```python
from build123d import *

# Parameters (mm, degrees)
PAD_DEPTH       = 250
SKETCH001_R     = 1.5
POCKET_DEPTH    = 10
SKETCH002_R     = 1.5
POCKET001_DEPTH = 10


with BuildPart() as part:
    # Sketch → Pad (new body)
    with BuildSketch(Plane.YZ):
        with BuildLine():
            Line((0, 0), (14, 0))
            Line((14, 0), (14, 1.524))
            Line((14, 1.524), (15.121, 1.524))
            Line((15.121, 1.524), (15.121, 7.862))
            ThreePointArc((15.121, 7.862), (8.692711, 6.292749), (2.787425, 3.307276))
            Line((0.963795, 6), (2.787425, 3.307276))
            Line((0, 6), (0.963795, 6))
            Line((0, 0), (0, 6))
        make_face()
    extrude(amount=PAD_DEPTH)

    # Sketch001 (on Face10 of Pad) → Pocket (cut)
    with BuildSketch(Plane.YZ.offset(250)):
        with Locations((12, 4)):
            Circle(SKETCH001_R)
        with Locations((5, 2)):
            Circle(SKETCH001_R)
    extrude(amount=-POCKET_DEPTH, mode=Mode.SUBTRACT)

    # Sketch002 (on Face4 of Pocket) → Pocket001 (cut)
    with BuildSketch(Plane(origin=(0, 0, 0), x_dir=(0, 1, 0), z_dir=(-1, 0, 0))):
        with Locations((12, -4)):
            Circle(SKETCH002_R)
        with Locations((5, -2)):
            Circle(SKETCH002_R)
    extrude(amount=-POCKET001_DEPTH, mode=Mode.SUBTRACT)


solid = part.part
```
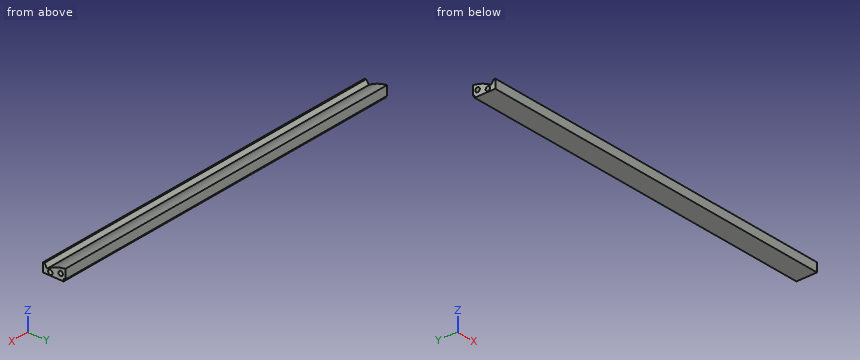
Work out the finished part from the listing and answer in its coordinate system (mm). Give positions to 0.01 mm unless a question says otherwise; leave off trailing zeros. Order: outer loops, then holes, each group sorted by start corner. A loop starts at its lowest first (then second) coordinate and runs counter-clockwise, first axis right, second up. Notation, with made-up numbers: M -3.75,25.5 L 3.25,25.5 A29 ccw 3.25,61.5 Z; hole C 18,-33 d4. An arc over 180 degrees is marked long. Return JSON: item names as keys, results as strings.
1) Straight lines are drawn through the part: line 1 along Y through (x, z) = (8.25, 2); line 2 along Y through (x, z) = (4.75, 4); line 3 along Z through (x, y) = (245.5, 5). For each, find the intervals that lie inside material, in ascending order. Write a range as [from, to].
Resolved:
{"line 1": "[0, 3.5], [6.5, 15.12]", "line 2": "[0, 2.32], [3.89, 10.5], [13.5, 15.12]", "line 3": "[0, 0.5], [3.5, 4.63]"}
2) Section A-A, the plane x = 148 is taken. Write down the section's boundary in (y, z), plus the area to 3 significant figures.
Resolved:
{"outline": "M 0,0 L 14,0 L 14,1.52 L 15.12,1.52 L 15.12,7.86 A29 ccw 2.79,3.31 L 0.96,6 L 0,6 Z", "area": "88.1 mm^2"}
3) Each of these flat-tipped pins is pushed along its axis until it touches: pin 1 (1.5 mm diameter, centred on y = 4.5, z = 2, fed in from +X); pin 2 (1.1 mm diameter, centred on x = 120.5, y = 0.5, fed in from +Z); pin 3 (8 mm diameter, centred on x = 168, y = 7, fed in from +Z). Where does it stop, or does it pass through?
Resolved:
{"pin 1": "x = 240", "pin 2": "z = 6", "pin 3": "z = 7.04"}
